Read the model definition and answer for the solid it produces. Units are mm, in the model's axes. A direction names the side the tool comes from. Round coordinates to 2 decimals unless told otherwise and drop trailing zeros. Write each loop counter-clockwise with the first axis right and the second up, starting at its lowest first coordinate (ties: lowest second). Pieces come first, ordered by that corner, then holes. Notation, with made-up numbers: (44, -28.5) - (94, -28.5) arc R22 cw to (94, -13.5) - close; hole circle Ø4 at (-24.5, -4). An arc over 180 degrees is marked (long way). One line per item, written item: value. Start each with the question number.
(1) A cutting plane is placed at C-C, the plane z = 130. Determine the outline of the cut face in (x, y).
(2) Find the intervals of material crossed by L1, parallel to Z at x = 4, y = -5; L2, parallel to X at y = 0.5, z = 101; L3, parallel to Y at x = -0.5, z = 7.5, in increasing order.
(3) For faces 1 (the face through (0, 0, 0)), 2 (the face through (-0.59, 4.46, 74.13)), determine the directions among +Z, -Z, +X, -X, +Y, -Y from which every point of the face is accessible in a straight line to the end or side of a thin tool.
(4) The mould has two halves that part along Z. Classify faces 3 (the face through (0, 0, 150)), 4 (the face through (4.1, 2.2, 137)), 5 (the face through (-11.99, 0.53, 143.56)): +Z half, -Z half, draft (parallel to the pull), parting line (faces both ways), or undercut.
(5) Flat-ended cylindrical pins translate along their axes: pin 1 Ø8 at (x, z) = (-3, 25.5) entering from -Y; pin 2 Ø10 at (y, z) = (7.5, 72) entering from +X; pin 3 Ø6 at (x, z) = (4.5, 75) entering from +Y; pin 4 Ø6 at (x, z) = (-9, 44) entering from +Y. Find the tip coordinate at first contact, or state that the pin passes through.
(6) A cutting plane is placed at A-A, the plane y = 0. Determine the outline of the cut face in (x, z).
from build123d import *

# Parameters (mm, degrees)
F0_R     = 4.5
F1_DEPTH = 150
F0_R_2   = 12
F2_DEPTH = 13
F3_R     = 12
F4_DEPTH = 13
F5_R     = 2.5


with BuildPart() as f1:
    # F0 (on Top) → F1 (new body)
    with BuildSketch(Plane.XY):
        Circle(F0_R)
    extrude(amount=F1_DEPTH)

    # F0 (on Top) → F2 (join)
    with BuildSketch(Plane.XY):
        Circle(F0_R_2)
        Circle(F0_R, mode=Mode.SUBTRACT)
    extrude(amount=F2_DEPTH)

    # F3 (on face) → F4 (join)
    with BuildSketch(Plane.XY.offset(150)):
        Circle(F3_R)
    extrude(amount=-F4_DEPTH)

    # F5
    f5_edges = [f1.edges().sort_by_distance(p)[0] for p in [
        (-12, 0, 150),
        (-12, 0, 137),
        (-12, 0, 13),
        (-12, 0, 0),
    ]]
    fillet(f5_edges, radius=F5_R)


solid = f1.part
Here are the results:
1. outline: circle Ø9 at (0, 0)
2. L1: 0 to 13, 137 to 150
2. L2: -4.47 to 4.47
2. L3: -11.99 to 11.99
3. face 1: -Z, +X, -X, +Y, -Y
3. face 2: none
4. face 3: +Z half
4. face 4: undercut
4. face 5: draft
5. pin 1: y = -4.5
5. pin 2: x = 3.74
5. pin 3: y = 4.24
5. pin 4: through
6. outline: (-12, 2.5) arc R2.5 ccw to (-9.5, 0) - (9.5, 0) arc R2.5 ccw to (12, 2.5) - (12, 10.5) arc R2.5 ccw to (9.5, 13) - (4.5, 13) - (4.5, 137) - (9.5, 137) arc R2.5 ccw to (12, 139.5) - (12, 147.5) arc R2.5 ccw to (9.5, 150) - (-9.5, 150) arc R2.5 ccw to (-12, 147.5) - (-12, 139.5) arc R2.5 ccw to (-9.5, 137) - (-4.5, 137) - (-4.5, 13) - (-9.5, 13) arc R2.5 ccw to (-12, 10.5) - close
